Geometry check sheet. Reference: drawing and pictorial views, mm from the part's lowest x, y, z. Give positions to 0.01 mm unless a question says otherwise; leave off trailing zeros. Loops run counter-clockwise (first coordinate to the right, second up) from the corner with the lowest first, then second, coordinate; pieces in that order, holes last. Notation, with made-up numbers: (84.25, 38) - (112.25, 38) arc R23 ccw to (112.25, 70) - close; hole circle Ø3 at (-30.5, -20.5). An arc over 180 degrees is marked (long way). Answer in a Markdown table with one row per item. Add a question column.
(1) Thickness scan on L1, parallel to X at y = 4.75, z = 3; L2, parallel to X at y = 3.75, z = 31; L3, parallel to Y at x = 5.75, z = 54.5. Record the ranges inside material, lowest first.
(2) Sectioned sample at C-C on y = 6.5. Enter the section's corners in (x, z), then the cut area to 3 significant figures.
(3) Sectioned sample at B-B on x = 9. Enter the section's corners in (y, z).
(4) Go/stop test with flat-tipped pins: P1, Ø6, axis at y = 3, z = 38, coming from the +X side; P2, Ø2, axis at y = 8.5, z = 33, coming from the +X side; P3, Ø1, axis at y = 6, z = 8.5, coming from the -X side; P4, Ø1.5, axis at x = 7, z = 9.5, coming from the -Y side. Record where each tip stops, or that it passes through.
(5) Sectioned sample at A-A on z = 62. Enter the section's corners in (x, y), then the cut area to 3 significant figures.
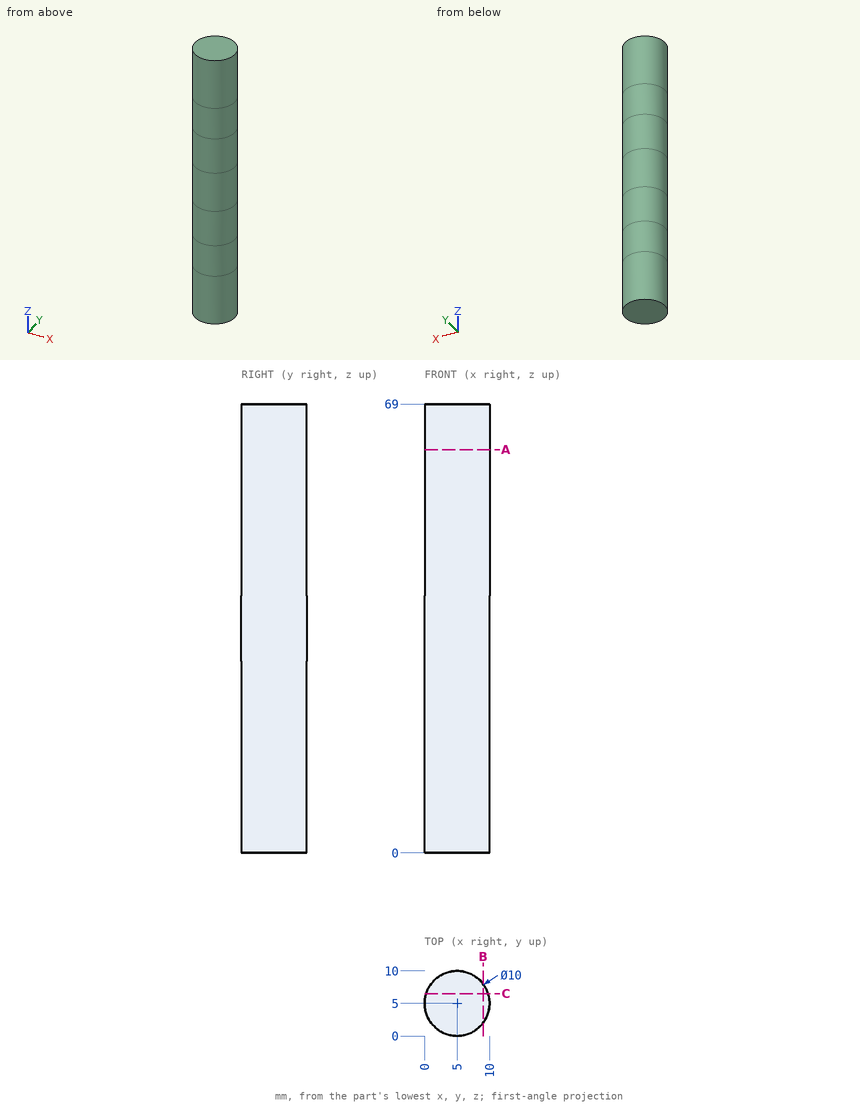
Reply:
| question | item | result |
|---|---|---|
| 1 | L1 | 0.01 to 9.99 |
| 1 | L2 | 0.16 to 9.84 |
| 1 | L3 | 0.06 to 9.94 |
| 2 | outline | (0.23, 0) - (9.77, 0) - (9.77, 69) - (0.23, 69) - close |
| 2 | area | 658 mm^2 |
| 3 | outline | (2, 0) - (8, 0) - (8, 69) - (2, 69) - close |
| 4 | P1 | x = 10 |
| 4 | P2 | x = 9.33 |
| 4 | P3 | x = 0.03 |
| 4 | P4 | y = 0.16 |
| 5 | outline | circle Ø10 at (5, 5) |
| 5 | area | 78.5 mm^2 |
